Here's how the part is built. I have some questions about the finished solid (model axes, mm). A direction names the side the tool comes from. Round coordinates to 2 decimals unless told otherwise and drop trailing zeros. Order: outer loops, then holes, each group sorted by start corner. A loop starts at its lowest first (then second) coordinate and runs counter-clockwise, first axis right, second up. Notation, with made-up numbers: (8, 23) - (45, 23) arc R30 ccw to (45, 48) - close; hole circle Ø5 at (33.25, -16.5). An arc over 180 degrees is marked (long way). Answer as a JSON object with one key per item and string values.
```python
from build123d import *

# Parameters (mm, degrees)
SZKIC2_R                    = 3.4
DODANIE_WYCI_GNI_CIE1_DEPTH = 84


with BuildPart() as part:
    # Szkic2 → Dodanie-wyciągnięcie1 (new body)
    with BuildSketch(Plane(origin=(0, 0, 0), x_dir=(1, 0, 0), z_dir=(0, 1, 0))):
        with BuildLine():
            Line((15.000219073, 4.001445911), (15.000219073, 13.001445911))
            ThreePointArc((15.000219073, 13.001445911), (14.414432635, 14.415659474), (13.000219073, 15.001445911))
            Line((13.000219073, 15.001445911), (4.000219073, 15.001445911))
            Line((4.000219073, 15.001445911), (4.000219073, 13.501445911))
            Line((4.000219073, 13.501445911), (8.500219073, 13.501445911))
            Line((8.500219073, 13.501445911), (8.500219073, 9.915659474))
            Line((8.500219073, 9.915659474), (4.38600551, 5.801445911))
            Line((4.38600551, 5.801445911), (-4.385567365, 5.801445911))
            Line((-4.385567365, 5.801445911), (-8.499780927, 9.915659474))
            Line((-8.499780927, 9.915659474), (-8.499780927, 13.501445911))
            Line((-8.499780927, 13.501445911), (-3.999780927, 13.501445911))
            Line((-3.999780927, 13.501445911), (-3.999780927, 15.001445911))
            Line((-3.999780927, 15.001445911), (-12.999780927, 15.001445911))
            ThreePointArc((-12.999780927, 15.001445911), (-14.41399449, 14.415659474), (-14.999780927, 13.001445911))
            Line((-14.999780927, 13.001445911), (-14.999780927, 4.001445911))
            Line((-14.999780927, 4.001445911), (-13.499780927, 4.001445911))
            Line((-13.499780927, 4.001445911), (-13.499780927, 8.501445911))
            Line((-13.499780927, 8.501445911), (-9.91399449, 8.501445911))
            Line((-9.91399449, 8.501445911), (-5.799780927, 4.387232349))
            Line((-5.799780927, 4.387232349), (-5.799780927, -4.384340526))
            Line((-5.799780927, -4.384340526), (-9.91399449, -8.498554089))
            Line((-9.91399449, -8.498554089), (-13.499780927, -8.498554089))
            Line((-13.499780927, -8.498554089), (-13.499780927, -3.998554089))
            Line((-13.499780927, -3.998554089), (-14.999780927, -3.998554089))
            Line((-14.999780927, -3.998554089), (-14.999780927, -12.998554089))
            ThreePointArc((-14.999780927, -12.998554089), (-14.41399449, -14.412767651), (-12.999780927, -14.998554089))
            Line((-12.999780927, -14.998554089), (-3.999780927, -14.998554089))
            Line((-3.999780927, -14.998554089), (-3.999780927, -13.498554089))
            Line((-3.999780927, -13.498554089), (-8.499780927, -13.498554089))
            Line((-8.499780927, -13.498554089), (-8.499780927, -9.912767651))
            Line((-8.499780927, -9.912767651), (-4.385567365, -5.798554089))
            Line((-4.385567365, -5.798554089), (4.38600551, -5.798554089))
            Line((4.38600551, -5.798554089), (8.500219073, -9.912767651))
            Line((8.500219073, -9.912767651), (8.500219073, -13.498554089))
            Line((8.500219073, -13.498554089), (4.000219073, -13.498554089))
            Line((4.000219073, -13.498554089), (4.000219073, -14.998554089))
            Line((4.000219073, -14.998554089), (13.000219073, -14.998554089))
            ThreePointArc((13.000219073, -14.998554089), (14.414432635, -14.412767651), (15.000219073, -12.998554089))
            Line((15.000219073, -12.998554089), (15.000219073, -3.998554089))
            Line((15.000219073, -3.998554089), (13.500219073, -3.998554089))
            Line((13.500219073, -3.998554089), (13.500219073, -8.498554089))
            Line((13.500219073, -8.498554089), (9.914432635, -8.498554089))
            Line((9.914432635, -8.498554089), (5.800219073, -4.384340526))
            Line((5.800219073, -4.384340526), (5.800219073, 4.387232349))
            Line((5.800219073, 4.387232349), (9.914432635, 8.501445911))
            Line((9.914432635, 8.501445911), (13.500219073, 8.501445911))
            Line((13.500219073, 8.501445911), (13.500219073, 4.001445911))
            Line((13.500219073, 4.001445911), (15.000219073, 4.001445911))
        make_face()
        with Locations(Location((0, 0, 0), (0, 0, 90))):
            Circle(SZKIC2_R, mode=Mode.SUBTRACT)
        with BuildLine():
            Line((10.001445911, -10.000219073), (13.501445911, -10.000219073))
            Line((13.501445911, -10.000219073), (13.501445911, -13.000219073))
            ThreePointArc((13.501445911, -13.000219073), (13.354999302, -13.353772463), (13.001445911, -13.500219073))
            Line((13.001445911, -13.500219073), (10.001445911, -13.500219073))
            Line((10.001445911, -13.500219073), (10.001445911, -10.000219073))
        make_face(mode=Mode.SUBTRACT)
        with BuildLine():
            Line((10.000219073, 10.001445911), (13.500219073, 10.001445911))
            Line((13.500219073, 10.001445911), (13.500219073, 13.001445911))
            ThreePointArc((13.500219073, 13.001445911), (13.353772463, 13.354999302), (13.000219073, 13.501445911))
            Line((13.000219073, 13.501445911), (10.000219073, 13.501445911))
            Line((10.000219073, 13.501445911), (10.000219073, 10.001445911))
        make_face(mode=Mode.SUBTRACT)
        with BuildLine():
            Line((-10.000219073, -10.001445911), (-10.000219073, -13.501445911))
            Line((-10.000219073, -13.501445911), (-13.000219073, -13.501445911))
            ThreePointArc((-13.000219073, -13.501445911), (-13.353772463, -13.354999302), (-13.500219073, -13.001445911))
            Line((-13.500219073, -13.001445911), (-13.500219073, -10.001445911))
            Line((-13.500219073, -10.001445911), (-10.000219073, -10.001445911))
        make_face(mode=Mode.SUBTRACT)
        with BuildLine():
            Line((-10.001445911, 10.000219073), (-13.501445911, 10.000219073))
            Line((-13.501445911, 10.000219073), (-13.501445911, 13.000219073))
            ThreePointArc((-13.501445911, 13.000219073), (-13.354999302, 13.353772463), (-13.001445911, 13.500219073))
            Line((-13.001445911, 13.500219073), (-10.001445911, 13.500219073))
            Line((-10.001445911, 13.500219073), (-10.001445911, 10.000219073))
        make_face(mode=Mode.SUBTRACT)
    extrude(amount=DODANIE_WYCI_GNI_CIE1_DEPTH)


solid = part.part
```
1. For faces 4 (the face through (9, 41, -15.001)), 5 (the face through (-14, 41, 3.999)), 6 (the face through (8.5, 41, -12)), 7 (the face through (4, 41, 14)), which set-ups out of +Z, -Z, +X, -X, +Y, -Y let a thin tool reach every point of the face, with its end or its side?
Responses:
{"face 4": "-Z, +X, -X, +Y, -Y", "face 5": "-X, +Y, -Y", "face 6": "+Y, -Y", "face 7": "+Z, +Y, -Y"}
2. For P1, Ø1.6, axis at x = -14.5, y = 51.5, coming from the +Z side; P2, Ø1.2, axis at x = 14.5, y = 54.5, coming from the -Z side; P3, Ø1.2, axis at y = 52.5, z = -14, coming from the -X side, each with a flat end and sliding along its axis, tell me the tip position at first contact or that it passes through.
Responses:
{"P1": "z = 14.87", "P2": "z = -14.79", "P3": "x = -14.96"}
3. Imagine slicing it at B-B (x = 11). List the corners of the cut face in (y, z) for me, plus the area to 3 significant figures.
Responses:
{"outline": "(0, -15) - (84, -15) - (84, -13.5) - (0, -13.5) - close; (0, -10) - (84, -10) - (84, -8.5) - (0, -8.5) - close; (0, 8.5) - (84, 8.5) - (84, 10) - (0, 10) - close; (0, 13.5) - (84, 13.5) - (84, 15) - (0, 15) - close", "area": "504 mm2"}
4. Imagine slicing it at C-C (x = 0). List the corners of the cut face in (y, z) for me.
Responses:
{"outline": "(0, -5.8) - (84, -5.8) - (84, -3.4) - (0, -3.4) - close; (0, 3.4) - (84, 3.4) - (84, 5.8) - (0, 5.8) - close"}
5. Imagine slicing it at A-A (z = 0). List the corners of the cut face in (x, y) for me, plus the area to 3 significant figures.
Responses:
{"outline": "(-5.8, 0) - (-3.4, 0) - (-3.4, 84) - (-5.8, 84) - close; (3.4, 0) - (5.8, 0) - (5.8, 84) - (3.4, 84) - close", "area": "403 mm2"}
6. If I drill on L1, parallel to X at y = 65, z = -11; L2, parallel to X at y = 29, z = -4.25, over which ranges is the centre line in solid material (lowest first)? Write a range as [from, to].
Responses:
{"L1": "[-15, -13.5], [-10, -8.5], [8.5, 10], [13.5, 15]", "L2": "[-15, -13.5], [-5.8, 5.8], [13.5, 15]"}
7. Thinking about a two-plate mould opening in X: for faces 1 (the face through (14, 41, 3.999)), 2 (the face through (6.472, 41.412, -7.887)), 3 (the face through (15, 41, 9)), which applies, pulls with the +X half, pulls with the -X half, needs draft (parallel to the pull), parting line crosses it, or undercut?
Responses:
{"face 1": "needs draft", "face 2": "undercut", "face 3": "pulls with the +X half"}
8. Imagine slicing it at D-D (z = -7.25). List the corners of the cut face in (x, y) for me, plus the area to 3 significant figures.
Responses:
{"outline": "(-15, 0) - (-13.5, 0) - (-13.5, 84) - (-15, 84) - close; (-8.66, 0) - (-5.83, 0) - (-5.83, 84) - (-8.66, 84) - close; (5.83, 0) - (8.66, 0) - (8.66, 84) - (5.83, 84) - close; (13.5, 0) - (15, 0) - (15, 84) - (13.5, 84) - close", "area": "727 mm2"}
